from build123d import *

# Parameters (mm, degrees)
F1_DEPTH = 12.7


with BuildPart() as f1:
    # F0 (on Front) → F1 (new body)
    with BuildSketch(Plane.XZ):
        with BuildLine():
            add(Edge.make_bspline(
                [(-38.6931858957, 54.3991737068), (-35.8405403413, 50.0610999657), (-32.9878947868, 45.7230262247), (-31.5682335133, 41.0291340153)],
                knots=[0, 0, 0, 0, 0.2439114114, 0.2439114114, 0.2439114114, 0.2439114114], degree=3))
            ThreePointArc((-38.6931858957, 54.3991737068), (-49.6350522053, 21.0007464247), (-26.8898194638, -5.7916736001))
            ThreePointArc((-26.8898194638, -5.7916736001), (-17.3939863098, -21.3085690308), (-0.2898975187, -27.5049419798))
            Line((-0.2898975187, -27.5049419798), (0.0159435843, 27.5064650525))
            ThreePointArc((0.0159435843, 27.5064650525), (-19.4983805085, 19.401521369), (-27.5060445831, -0.1529224477))
            add(Edge.make_bspline(
                [(-30.6462217122, 34.7148962319), (-30.7754650722, 27.1593597), (-39.1689548904, 11.6131795075), (-31.0760950053, 3.448715235), (-27.5060445831, -0.1529224477)],
                knots=[0.3493301375, 0.3493301375, 0.3493301375, 0.3493301375, 0.7129662134, 1, 1, 1, 1], degree=3))
            add(Edge.make_bspline(
                [(-31.5682335133, 41.0291340153), (-35.3674367785, 36.1399617518), (-42.4430865557, 27.1135638958), (-34.3396168251, 32.3313583593), (-30.6462217122, 34.7148962319)],
                knots=[0, 0, 0, 0, 0.5426319314, 1, 1, 1, 1], degree=3))
        make_face()
    extrude(amount=F1_DEPTH)

    # F2: F1 across plane


with BuildPart() as f1_1:
    add(f1.part)
    add(f1.part.mirror(Plane.YZ))


solid = f1_1.part
Here's how the part is built. I have some questions about the finished solid (model axes, mm). Coordinates: 2 decimals unless noted, no trailing zeros. Loops run counter-clockwise (first coordinate to the right, second up) from the corner with the lowest first, then second, coordinate; pieces in that order, holes last. Notation, with made-up numbers: (-38, 10.25) -> (-17, 10.25) arc R8 cw to (-17, 15.25) -> close; hole circle Ø6 at (-18.5, 77.25). An arc over 180 degrees is marked (long way). Use one line per item in the form item = value. Start each with the question number.
(1) Please list where these lines run through material, in increasing order: line 1 along X through (y, z) = (-6.5, 25); line 2 along X through (y, z) = (-5.25, 1); line 3 along X through (y, z) = (-9.75, 39).
(2) If we section it at C-C (x = 5): Please give me the cut outline in (y, z).
(3) If we section it at A-A (z = -18.5): Please give me the cut outline in (x, y), then the cut area to 3 significant figures.
(4) If we section it at B-B (z = -7): Please give me the cut outline in (x, y), then the cut area to 3 significant figures.
(5) Will these pins go through, and if not, where does the flat tip stop? pin 1 (6 mm diameter, centred on y = -3, z = 1, fed in from -X); pin 2 (2 mm diameter, centred on y = -8.5, z = 3.5, fed in from +X); pin 3 (6 mm diameter, centred on x = -11, y = -8, fed in from -Z).
(6) If we section it at D-D (z = 10.5): Give the number of separate pieces and of enclosed holes in the cut face, then the cut area to 3 significant figures.
Verdict:
q1.line_1 = -50.19 to -32.46, -11.47 to 11.47, 32.46 to 50.19
q1.line_2 = -38.19 to -28.64, -27.49 to -0.13, 0.13 to 27.49, 28.64 to 38.19
q1.line_3 = -48.56 to -33.14, 33.14 to 48.56
q2.outline = (-12.7, -27.05) -> (0, -27.05) -> (0, 27.05) -> (-12.7, 27.05) -> close
q3.outline = (-20.36, -12.7) -> (-0.24, -12.7) -> (-0.24, 0) -> (-20.36, 0) -> close; (0.24, -12.7) -> (20.36, -12.7) -> (20.36, 0) -> (0.24, 0) -> close
q3.area = 511 mm²
q4.outline = (-26.6, -12.7) -> (-0.18, -12.7) -> (-0.18, 0) -> (-26.6, 0) -> close; (0.18, -12.7) -> (26.6, -12.7) -> (26.6, 0) -> (0.18, 0) -> close
q4.area = 671 mm²
q5.pin_1 = -41.2
q5.pin_2 = 41.64
q5.pin_3 = -26.32
q6.separate_pieces = 4
q6.enclosed_holes = 0
q6.area = 924 mm²
